```python
from build123d import *

# Parameters (mm, degrees)
SKICA1_W                = 220
SKICA1_H                = 65
SKICA1_W_2              = 200
SKICA1_H_2              = 5
P_IDAT_VYSUNUT_M1_DEPTH = 35
P_IDAT_VYSUNUT_M2_DEPTH = 15


with BuildPart() as part:
    # Skica1 → Přidat vysunutím1 (new body)
    with BuildSketch(Plane(origin=(0, 0, 0), x_dir=(1, 0, 0), z_dir=(0, 1, 0))):
        with Locations((110, 32.5)):
            Rectangle(SKICA1_W, SKICA1_H)
        with Locations((110, 32.5)):
            Rectangle(SKICA1_W_2, SKICA1_H_2, mode=Mode.SUBTRACT)
    extrude(amount=P_IDAT_VYSUNUT_M1_DEPTH)

    # Skica2 → Přidat vysunutím2 (add)
    with BuildSketch(Plane(origin=(0, 35, 0), x_dir=(1, 0, 0), z_dir=(0, 1, 0))):
        Polygon((15, 15), (15, 19), (20.5, 19), (20.5, 24.5), (24.5, 24.5), (24.5, 19), (30, 19), (30, 15), (24.5, 15), (24.5, 9.5), (20.5, 9.5), (20.5, 15), align=None)
        Polygon((24.5, 50), (30, 50), (30, 46), (24.5, 46), (24.5, 40.5), (20.5, 40.5), (20.5, 46), (15, 46), (15, 50), (20.5, 50), (20.5, 55.5), (24.5, 55.5), align=None)
        Polygon((205, 50), (205, 46), (199.5, 46), (199.5, 40.5), (195.5, 40.5), (195.5, 46), (190, 46), (190, 50), (195.5, 50), (195.5, 55.5), (199.5, 55.5), (199.5, 50), align=None)
        Polygon((205, 15), (199.5, 15), (199.5, 9.5), (195.5, 9.5), (195.5, 15), (190, 15), (190, 19), (195.5, 19), (195.5, 24.5), (199.5, 24.5), (199.5, 19), (205, 19), align=None)
    extrude(amount=P_IDAT_VYSUNUT_M2_DEPTH)


solid = part.part
```
Here's how the part is built. I have some questions about the finished solid (model axes, mm). A direction names the side the tool comes from. Round coordinates to 2 decimals unless told otherwise and drop trailing zeros. Order: outer loops, then holes, each group sorted by start corner. A loop starts at its lowest first (then second) coordinate and runs counter-clockwise, first axis right, second up. Notation, with made-up numbers: (27, 74) -> (54, 74) arc R22 cw to (54, 112) -> close; hole circle Ø6 at (83, 13). An arc over 180 degrees is marked (long way). Use a Markdown table: item, result. Add a question column.
(1) Suppose I cut it at D-D, the plane z = -52. Please give me the cut outline in (x, y), and give its area (3 significant figures).
(2) I need wall thicknesses on line 1 along Z through (x, y) = (71, 22.5); line 2 along Z through (x, y) = (17, 38); line 3 along X through (y, z) = (37.5, -53). Which ranges of each line are inside material? Lowest first, please.
(3) Suppose I cut it at B-B, the plane z = -33. Please give me the cut outline in (x, y).
(4) Suppose I cut it at A-A, the plane x = 123. Please give me the cut outline in (y, z).
(5) If we mould it in two halves opening along X, with no side actions, what happens to faces 6 (the face through (195.5, 42, -12)), 7 (the face through (20.5, 42, -22)), 8 (the face through (108, 0, -40))? For each: released by +X, released by -X, zero draft, split by the parting line, or undercut.
(6) For pin 1 Ø1.6 at (y, z) = (42.5, -53.5) entering from +X; pin 2 Ø1.6 at (x, y) = (16.5, 45.5) entering from +Z; pin 3 Ø2 at (y, z) = (41.5, -47) entering from -X, each with a flat end and sliding along its axis, tell me the tip position at first contact or that it passes through.
(7) Suppose I cut it at C-C, the plane y = 18. Please give me the cut outline in (x, z).
(8) For faces 1 (the face through (190, 42, -48)), 2 (the face through (10, 17, -32)), 3 (the face through (193, 42, -50)), 4 (the face through (193, 42, -46)), 5 (the face through (18, 42, -50)), which set-ups out of +Z, -Z, +X, -X, +Y, -Y let a thin tool reach every point of the face, with its end or its side?
Verdict:
| question | item | result |
|---|---|---|
| 1 | outline | (0, 0) -> (220, 0) -> (220, 35) -> (199.5, 35) -> (199.5, 50) -> (195.5, 50) -> (195.5, 35) -> (24.5, 35) -> (24.5, 50) -> (20.5, 50) -> (20.5, 35) -> (0, 35) -> close |
| 1 | area | 7,820 mm2 |
| 2 | line 1 | -65 to -35, -30 to 0 |
| 2 | line 2 | -50 to -46, -19 to -15 |
| 2 | line 3 | 20.5 to 24.5, 195.5 to 199.5 |
| 3 | outline | (0, 0) -> (10, 0) -> (10, 35) -> (0, 35) -> close; (210, 0) -> (220, 0) -> (220, 35) -> (210, 35) -> close |
| 4 | outline | (0, -65) -> (35, -65) -> (35, -35) -> (0, -35) -> close; (0, -30) -> (35, -30) -> (35, 0) -> (0, 0) -> close |
| 5 | face 6 | undercut |
| 5 | face 7 | released by -X |
| 5 | face 8 | zero draft |
| 6 | pin 1 | x = 199.5 |
| 6 | pin 2 | z = -15 |
| 6 | pin 3 | x = 15 |
| 7 | outline | (0, -65) -> (220, -65) -> (220, 0) -> (0, 0) -> close; hole (10, -35) -> (210, -35) -> (210, -30) -> (10, -30) -> close |
| 8 | face 1 | +Z, -Z, +Y |
| 8 | face 2 | +Y, -Y |
| 8 | face 3 | -Z, +Y |
| 8 | face 4 | +Y |
| 8 | face 5 | -Z, -X, +Y |
